Could you check a few things on this model? Use its own coordinates, in mm. Face numbers are marked on the shaded views. A direction names the side the tool comes from. Round coordinates to 2 decimals unless told otherwise and drop trailing zeros. Loops run counter-clockwise (first coordinate to the right, second up) from the corner with the lowest first, then second, coordinate; pieces in that order, holes last. Notation, with made-up numbers: (60.25, 13) -> (91.25, 13) arc R13 cw to (91.25, 33) -> close; hole circle Ø10 at (46.25, 34.5). An arc over 180 degrees is marked (long way). Write each question's results on one line, items separated by ' | '.
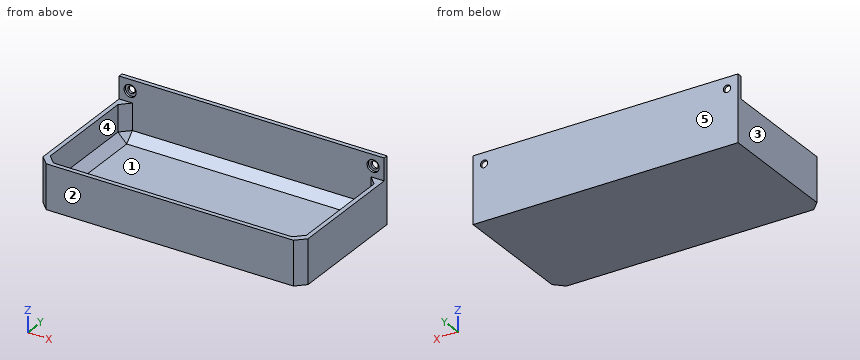
from build123d import *

# Parameters (mm, degrees)
F0_W     = 152.4
F0_H     = 76.2
F0_W_2   = 147.32
F0_H_2   = 71.12
F1_DEPTH = 25.4
F2_DEPTH = 5.08
F4_DEPTH = 12.7
F5_R     = 3.4925
F5_R_2   = 2.0955
F6_DEPTH = 1.27
F7_DEPTH = 25.4
F8_SIZE  = 5.08


with BuildPart() as f1:
    # F0 (on Top) → F1 (new body)
    with BuildSketch(Plane.XY):
        with Locations((76.2, 38.1)):
            Rectangle(F0_W, F0_H)
        with Locations((76.2, 38.1)):
            Rectangle(F0_W_2, F0_H_2, mode=Mode.SUBTRACT)
    extrude(amount=F1_DEPTH)

    # F0 (on Top) → F2 (join)
    with BuildSketch(Plane.XY):
        with Locations((76.2, 38.1)):
            Rectangle(F0_W, F0_H)
        with Locations((76.2, 38.1)):
            Rectangle(F0_W_2, F0_H_2, mode=Mode.SUBTRACT)
        with Locations((76.2, 38.1)):
            Rectangle(F0_W_2, F0_H_2)
    extrude(amount=F2_DEPTH)

    # F3 (on face) → F4 (join)
    with BuildSketch(Plane.XY.offset(25.4)):
        Polygon((0, 76.2), (0, 73.66), (2.54, 73.66), (149.86, 73.66), (152.4, 73.66), (152.4, 76.2), align=None)
    extrude(amount=F4_DEPTH)

    # F5 (on face) → F6 (cut)
    with BuildSketch(Plane.XZ.offset(-73.66)):
        with Locations((6.35, 31.75)):
            Circle(F5_R)
        with Locations((6.35, 31.75)):
            Circle(F5_R_2, mode=Mode.SUBTRACT)
        with Locations((146.05, 31.75)):
            Circle(F5_R)
        with Locations((146.05, 31.75)):
            Circle(F5_R_2, mode=Mode.SUBTRACT)
    extrude(amount=-F6_DEPTH, mode=Mode.SUBTRACT)

    # F7 (cut): faces of the model
    f7_faces = [f1.faces().sort_by_distance(p)[0] for p in [
        (6.35, 73.66, 31.75),
        (146.05, 73.66, 31.75),
    ]]
    extrude(f7_faces, amount=-F7_DEPTH, mode=Mode.SUBTRACT)

    # F8
    f8_edges = [f1.edges().sort_by_distance(p)[0] for p in [
        (2.54, 73.66, 15.24),
        (76.2, 73.66, 5.08),
        (2.54, 38.1, 5.08),
        (76.2, 2.54, 5.08),
        (149.86, 38.1, 5.08),
        (2.54, 2.54, 15.24),
        (149.86, 2.54, 15.24),
        (149.86, 73.66, 15.24),
        (0, 0, 12.7),
        (152.4, 0, 12.7),
    ]]
    chamfer(f8_edges, length=F8_SIZE)


solid = f1.part
1) If we mould it in two halves opening along X, with no side actions, what happens to the marked faces 1, 2 and 3? For each: released by +X, released by -X, zero draft, split by the parting line, or undercut.
Model answer:
face 1: undercut | face 2: zero draft | face 3: released by -X
2) I want a section at D-D, the plane x = 74. Write out the boundary of the cut face in (y, z), plus the area to 3 significant figures.
Model answer:
outline: (0, 0) -> (76.2, 0) -> (76.2, 38.1) -> (73.66, 38.1) -> (73.66, 10.16) -> (68.58, 5.08) -> (7.62, 5.08) -> (2.54, 10.16) -> (2.54, 25.4) -> (0, 25.4) -> close | area: 548 mm2
3) I want a section at C-C, the plane y = 64.5. Write out the boundary of the cut face in (x, z), plus the area to 3 significant figures.
Model answer:
outline: (0, 0) -> (152.4, 0) -> (152.4, 25.4) -> (149.86, 25.4) -> (149.86, 10.16) -> (144.78, 5.08) -> (7.62, 5.08) -> (2.54, 10.16) -> (2.54, 25.4) -> (0, 25.4) -> close | area: 903 mm2
4) I want a section at B-B, the plane z = 31.75. Write out the boundary of the cut face in (x, y).
Model answer:
outline: (0, 73.66) -> (2.86, 73.66) -> (2.86, 74.93) -> (4.25, 74.93) -> (4.25, 76.2) -> (0, 76.2) -> close; (8.45, 74.93) -> (9.84, 74.93) -> (9.84, 73.66) -> (142.56, 73.66) -> (142.56, 74.93) -> (143.95, 74.93) -> (143.95, 76.2) -> (8.45, 76.2) -> close; (148.15, 74.93) -> (149.54, 74.93) -> (149.54, 73.66) -> (152.4, 73.66) -> (152.4, 76.2) -> (148.15, 76.2) -> close
5) For the marked faces 4 and 5, which set-ups out of +Z, -Z, +X, -X, +Y, -Y let a thin tool reach every point of the face, with its end or its side?
Model answer:
face 4: +Z | face 5: +Z, -Z, +X, -X, +Y
6) I want a section at A-A, the plane z = 21. Write out the boundary of the cut face in (x, y).
Model answer:
outline: (0, 5.08) -> (5.08, 0) -> (147.32, 0) -> (152.4, 5.08) -> (152.4, 76.2) -> (0, 76.2) -> close; hole (2.54, 7.62) -> (7.62, 2.54) -> (144.78, 2.54) -> (149.86, 7.62) -> (149.86, 68.58) -> (144.78, 73.66) -> (7.62, 73.66) -> (2.54, 68.58) -> close
7) I need wall thicknesses on line 1 (Y direction, x = 130.5, z = 19); line 2 (X direction, y = 47, z = 16.5); line 3 (Z direction, x = 146, y = 75). Which ranges of each line are inside material? Lowest first, please.
Model answer:
line 1: y = 0 to 2.54, 73.66 to 76.2 | line 2: x = 0 to 2.54, 149.86 to 152.4 | line 3: z = 0 to 29.66, 33.84 to 38.1
8) I'm going to push flat-ended pins straight in: pin 1 (5 mm diameter, centred on x = 113, y = 35, fed in from +Z); pin 2 (7.5 mm diameter, centred on x = 147.5, z = 33.5, fed in from -Y); pin 3 (4 mm diameter, centred on x = 6.35, z = 31.75, fed in from +Y); pin 4 (2 mm diameter, centred on x = 5, z = 30, fed in from -Y). Where does each tip first touch, or does it pass through?
Model answer:
pin 1: stops at z = 5.08 | pin 2: stops at y = 73.66 | pin 3: passes through | pin 4: stops at y = 74.93
